For this review, take the finished solid that the model builds, in its own axes (mm). Give positions to 0.01 mm unless a question says otherwise; leave off trailing zeros. Loops run counter-clockwise (first coordinate to the right, second up) from the corner with the lowest first, then second, coordinate; pieces in that order, holes last. Notation, with made-up numbers: (-16.5, 28.5) - (18.5, 28.5) arc R17 cw to (18.5, 50.5) - close; hole circle Ø5 at (-32.5, -14.5). An arc over 180 degrees is marked (long way). Put each result on its own line as item: value.
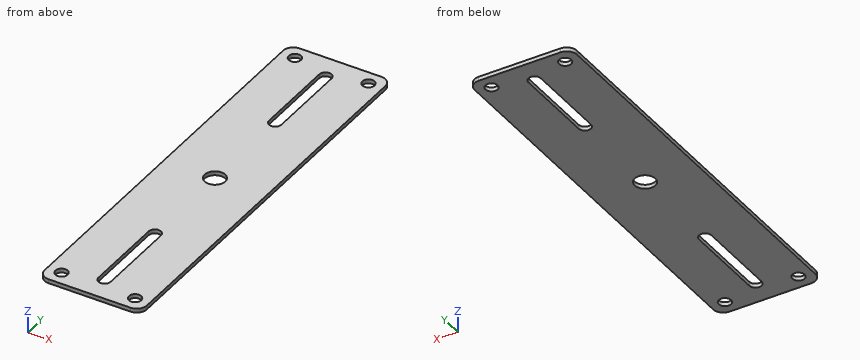
from build123d import *

# Parameters (mm, degrees)
SCHIZZO1_W                   = 50
SCHIZZO1_H                   = 100
SCHIZZO1_R                   = 3
ESTRUSIONE_ESTRUSIONE1_DEPTH = 2
RACCORDO3_R                  = 5
RACCORDO4_R                  = 5
SCHIZZO3_R                   = 5
TAGLIO_ESTRUSIONE1_DEPTH     = 104.097041665


with BuildPart() as part:
    # Schizzo1 → Estrusione-Estrusione1 (new body)
    with BuildSketch(Plane.XY):
        with Locations((0, 50)):
            Rectangle(SCHIZZO1_W, SCHIZZO1_H)
        with Locations((-18, 93)):
            Circle(SCHIZZO1_R, mode=Mode.SUBTRACT)
        with Locations((18, 93)):
            Circle(SCHIZZO1_R, mode=Mode.SUBTRACT)
        with BuildLine():
            Line((-3, 88), (-3, 48))
            ThreePointArc((-3, 48), (0, 45), (3, 48))
            Line((3, 48), (3, 88))
            ThreePointArc((3, 88), (0, 91), (-3, 88))
        make_face(mode=Mode.SUBTRACT)
    extrude(amount=ESTRUSIONE_ESTRUSIONE1_DEPTH)

    # Raccordo3
    raccordo3_edges = [part.edges().sort_by_distance(p)[0] for p in [
        (25, 100, 1),
    ]]
    fillet(raccordo3_edges, radius=RACCORDO3_R)

    # Raccordo4
    raccordo4_edges = [part.edges().sort_by_distance(p)[0] for p in [
        (-25, 100, 1),
    ]]
    fillet(raccordo4_edges, radius=RACCORDO4_R)

    # Specchia1: part across plane


with BuildPart() as part_1:
    add(part.part)
    add(part.part.mirror(Plane(origin=(-25, 0, 2), x_dir=(0, 0, 1), z_dir=(0, 1, 0))))

    # Schizzo3 → Taglio-Estrusione1 (cut, through all)
    with BuildSketch(Plane.XY.offset(2)):
        Circle(SCHIZZO3_R)
    extrude(amount=-TAGLIO_ESTRUSIONE1_DEPTH, mode=Mode.SUBTRACT)


solid = part_1.part
1) Wall thickness on line 1 (Y direction, x = 18, z = 1); line 2 (X direction, y = -93, z = 0.4); line 3 (Y direction, x = 0, z = 0.6): over which ranges is each line inside the solid? List them lowest first.
Geometry check:
line 1: y = -100 to -96, -90 to 90, 96 to 100
line 2: x = -25 to -21, -15 to 15, 21 to 25
line 3: y = -100 to -91, -45 to -5, 5 to 45, 91 to 100
2) Insertion check: pin 1 Ø9.5 at (x, y) = (-18, 93) entering from +Z. The pin has a flat end and moves straight along its axis. Give the tip position at first contact, or say it passes through.
Geometry check:
pin 1: stops at z = 2
3) Take a section at C-C on y = -67. State the section outline as (x, z) points, and give its area (3 significant figures).
Geometry check:
outline: (-25, 0) - (-3, 0) - (-3, 2) - (-25, 2) - close; (3, 0) - (25, 0) - (25, 2) - (3, 2) - close
area: 88.0 mm²
4) Take a section at A-A on x = 0. State the section outline as (y, z) points.
Geometry check:
outline: (-100, 0) - (-91, 0) - (-91, 2) - (-100, 2) - close; (-45, 0) - (-5, 0) - (-5, 2) - (-45, 2) - close; (5, 0) - (45, 0) - (45, 2) - (5, 2) - close; (91, 0) - (100, 0) - (100, 2) - (91, 2) - close
5) Take a section at D-D on x = 18. State the section outline as (y, z) points, and give its area (3 significant figures).
Geometry check:
outline: (-100, 0) - (-96, 0) - (-96, 2) - (-100, 2) - close; (-90, 0) - (90, 0) - (90, 2) - (-90, 2) - close; (96, 0) - (100, 0) - (100, 2) - (96, 2) - close
area: 376 mm²
6) Take a section at B-B on z = 1.2. State the section outline as (x, y) points, and give its area (3 significant figures).
Geometry check:
outline: (-25, -95) arc R5 ccw to (-20, -100) - (20, -100) arc R5 ccw to (25, -95) - (25, 95) arc R5 ccw to (20, 100) - (-20, 100) arc R5 ccw to (-25, 95) - close; hole circle Ø6 at (-18, -93); hole circle Ø6 at (-18, 93); hole circle Ø10 at (0, 0); hole (-3, -88) arc R3 ccw to (3, -88) - (3, -48) arc R3 ccw to (-3, -48) - close; hole (-3, 48) arc R3 ccw to (3, 48) - (3, 88) arc R3 ccw to (-3, 88) - close; hole circle Ø6 at (18, -93); hole circle Ø6 at (18, 93)
area: 9,250 mm²
